Source: CAD feature listing. Evaluate the final solid. Frame: model axes, mm. A direction names the side the tool comes from. Give positions to 0.01 mm unless a question says otherwise; leave off trailing zeros. Order: outer loops, then holes, each group sorted by start corner. A loop starts at its lowest first (then second) coordinate and runs counter-clockwise, first axis right, second up. Notation, with made-up numbers: (-28.5, 50.25) -> (-2.5, 50.25) arc R28 cw to (-2.5, 72.25) -> close; hole circle Ø6 at (68.5, 77). An arc over 180 degrees is marked (long way). Answer in a Markdown table with one row per item.
```python
from build123d import *

# Parameters (mm, degrees)
F1_DEPTH  = 50.8
F2_W      = 15.9388422537
F2_H      = 34.29
F4_DEPTH  = 25.4
F3_W      = 26.67
F3_H      = 34.29
F5_DEPTH  = 25.4
F6_DEPTH  = 25.4
F7_W      = 15.9388422537
F7_H      = 34.29
F8_DEPTH  = 5.08
F9_R      = 4.6036191434
F10_DEPTH = 25.4
F12_DEPTH = 25.4


with BuildPart() as f1:
    # F0 (on Front) → F1 (new body)
    with BuildSketch(Plane.XZ):
        Polygon((0, -30.48), (0, 0), (-26.67, 0), (-26.67, 20.32), (-45.72, 20.32), (-45.72, -30.48), align=None)
    extrude(amount=-F1_DEPTH)

    # F2 (on face) → F4 (cut)
    with BuildSketch(Plane.XY.offset(20.32)):
        with Locations((-34.6394211268, 25.4)):
            Rectangle(F2_W, F2_H)
    extrude(amount=-F4_DEPTH, mode=Mode.SUBTRACT)

    # F3 (on face) → F5 (cut)
    with BuildSketch(Plane.XY):
        with Locations((-13.335, 25.4)):
            Rectangle(F3_W, F3_H)
    extrude(amount=-F5_DEPTH, mode=Mode.SUBTRACT)

    # F6 (cut): a face of the model
    f6_faces = [f1.faces().sort_by_distance(p)[0] for p in [
        (-34.6394211268, 25.4, -5.08),
    ]]
    extrude(f6_faces, amount=-F6_DEPTH, mode=Mode.SUBTRACT)

    # F7 (on face) → F8 (join)
    with BuildSketch(Plane(origin=(0, 0, -30.48), x_dir=(1, 0, 0), z_dir=(0, 0, -1))):
        with Locations((-34.6394211268, -25.4)):
            Rectangle(F7_W, F7_H)
    extrude(amount=-F8_DEPTH)

    # F9 (on face) → F10 (cut)
    with BuildSketch(Plane.YZ.offset(-42.6088422537)):
        with Locations((27.777671814, 1.571879955)):
            Circle(F9_R)
    extrude(amount=-F10_DEPTH, mode=Mode.SUBTRACT)

    # F11: F1 across face


with BuildPart() as f1_1:
    add(f1.part)
    add(f1.part.mirror(Plane(origin=(0, 25.4, -18.5057142857), x_dir=(0, 1, 0), z_dir=(1, 0, 0))))

    # F12 (cut): a face of the model
    f12_faces = [f1_1.faces().sort_by_distance(p)[0] for p in [
        (0, 25.4, -25.4),
    ]]
    extrude(f12_faces, amount=-F12_DEPTH, mode=Mode.SUBTRACT)


solid = f1_1.part
```
(1) Pull-direction query (Y, two-part tool) for faces 4 (the flat face through (1, 50.8, -10)), 5 (the flat face through (0, 47, 0)), 6 (the flat face through (1, 0, -10)), 7 (the flat face through (-42.609, 26, -5)); classes: +Y half, -Y half, draft (parallel to the pull), parting line (faces both ways), or undercut.
A:
| item | result |
|---|---|
| face 4 | +Y half |
| face 5 | draft |
| face 6 | -Y half |
| face 7 | undercut |
(2) Section query B-B (z = -20). Return the cut outline in (x, y) (3 decimals), plus the area to 3 significant figures.
A:
| item | result |
|---|---|
| outline | (-45.72, 0) -> (45.72, 0) -> (45.72, 50.8) -> (-45.72, 50.8) -> close; hole (-42.609, 8.255) -> (42.609, 8.255) -> (42.609, 42.545) -> (-42.609, 42.545) -> close |
| area | 1,720 mm^2 |
(3) Ray query, probe 1 along X at (y, z) = (2.5, 16.5); probe 2 along X at (y, z) = (22.5, 3); probe 3 along Y at (x, z) = (24, -2.5) (3 decimals). Return the intervals inside material, ascending.
A:
| item | result |
|---|---|
| probe 1 | x = -45.72 to -26.67, 26.67 to 45.72 |
| probe 2 | x = -45.72 to -42.61, 42.61 to 45.72 |
| probe 3 | y = 0 to 8.255, 42.545 to 50.8 |
(4) First-contact query: pin 1 Ø5.5 at (y, z) = (27.78, 1.57) entering from +X; pin 2 Ø4 at (x, y) = (-7, 2) entering from +Z; pin 3 Ø15 at (x, z) = (2, -15) entering from -Y. Flat tips, straight axial feed; report the tip coordinate or a pass-through.
A:
| item | result |
|---|---|
| pin 1 | passes through |
| pin 2 | stops at z = 0 |
| pin 3 | stops at y = 0 |
(5) Section query C-C (y = 36.5). Return the cut outline in (x, z).
A:
| item | result |
|---|---|
| outline | (-45.72, -30.48) -> (-42.61, -30.48) -> (-42.61, 20.32) -> (-45.72, 20.32) -> close; (42.61, -30.48) -> (45.72, -30.48) -> (45.72, 20.32) -> (42.61, 20.32) -> close |
(6) Access query for faces 1 (the flat face through (45, 19, 20.32)), 2 (the flat face through (-1, 42.545, -10)), 3 (the flat face through (-26.67, 47, 10)). Directions: +Z, -Z, +X, -X, +Y, -Y. A direction counts if a zero-diameter tool reaches every point of the face in a straight line with its end or side. Return the directions, or none.
A:
| item | result |
|---|---|
| face 1 | +Z, +X, -X, +Y, -Y |
| face 2 | +Z, -Z |
| face 3 | +Z, +Y, -Y |
(7) Section query A-A (x = -3). Return the cut outline in (y, z) (3 decimals), plus the area to 3 significant figures.
A:
| item | result |
|---|---|
| outline | (0, -30.48) -> (8.255, -30.48) -> (8.255, 0) -> (0, 0) -> close; (42.545, -30.48) -> (50.8, -30.48) -> (50.8, 0) -> (42.545, 0) -> close |
| area | 503 mm^2 |
(8) Section query D-D (z = 9). Return the cut outline in (x, y) (3 decimals), plus the area to 3 significant figures.
A:
| item | result |
|---|---|
| outline | (-45.72, 0) -> (-26.67, 0) -> (-26.67, 8.255) -> (-42.609, 8.255) -> (-42.609, 42.545) -> (-26.67, 42.545) -> (-26.67, 50.8) -> (-45.72, 50.8) -> close; (26.67, 0) -> (45.72, 0) -> (45.72, 50.8) -> (26.67, 50.8) -> (26.67, 42.545) -> (42.609, 42.545) -> (42.609, 8.255) -> (26.67, 8.255) -> close |
| area | 842 mm^2 |
